```python
from build123d import *

# Parameters (mm, degrees)
F0_W          = 15.24
F0_H          = 15.24
F1_DEPTH      = 35.56
F2_R          = 3.175
F3_DEPTH      = 12.7
F3_DEPTH_BACK = 3.175
F4_R          = 3.175
F4_W          = 11.2
F4_H          = 5.9
F5_DEPTH      = 12.7
F6_T1_DEPTH   = 48.26
F7_R          = 3.302
F8_DEPTH      = 6.35


# Not quite as in the source:
# - a fillet or chamfer that OpenCascade refuses, or shapes differently, is made with other operations: its cross-section is extruded or revolved along the edge and cut away or added


with BuildPart() as f1:
    # F0 (on Top) → F1 (new body)
    with BuildSketch(Plane.XY):
        Rectangle(F0_W, F0_H)
    extrude(amount=F1_DEPTH)

    # F2 (on Front) → F3 (cut, two sides)
    with BuildSketch(Plane.XZ) as f3_sk:
        with Locations((0, 34.00425)):
            Circle(F2_R)
    extrude(amount=-F3_DEPTH, mode=Mode.SUBTRACT)
    extrude(f3_sk.sketch, amount=F3_DEPTH_BACK, mode=Mode.SUBTRACT)

    # F4 (on Right) → F5 (cut, symmetric)
    with BuildSketch(Plane.YZ):
        with Locations((0, 25.4)):
            Circle(F4_R)
        with Locations((0, 6.35)):
            Rectangle(F4_W, F4_H)
    extrude(amount=F5_DEPTH, both=True, mode=Mode.SUBTRACT)

    # F6: fillet of radius 2.54 on 4 edges, made by hand

    # F6_s2 → F6_t1 (cut)
    with BuildSketch(Plane.XY.offset(-6.35)):
        with BuildLine():
            ThreePointArc((7.62, 5.08), (6.8760512242, 6.8760512242), (5.08, 7.62))
            Line((5.08, 7.62), (7.62, 7.62))
            Line((7.62, 7.62), (7.62, 5.08))
        make_face()
        with BuildLine():
            ThreePointArc((5.08, -7.62), (6.8760512242, -6.8760512242), (7.62, -5.08))
            Line((7.62, -5.08), (7.62, -7.62))
            Line((7.62, -7.62), (5.08, -7.62))
        make_face()
        with BuildLine():
            ThreePointArc((-7.62, 5.08), (-6.8760512242, 6.8760512242), (-5.08, 7.62))
            Line((-5.08, 7.62), (-7.62, 7.62))
            Line((-7.62, 7.62), (-7.62, 5.08))
        make_face()
        with BuildLine():
            ThreePointArc((-5.08, -7.62), (-6.8760512242, -6.8760512242), (-7.62, -5.08))
            Line((-7.62, -5.08), (-7.62, -7.62))
            Line((-7.62, -7.62), (-5.08, -7.62))
        make_face()
    extrude(amount=F6_T1_DEPTH, mode=Mode.SUBTRACT)

    # F7 (on face) → F8 (cut)
    with BuildSketch(Plane(origin=(0, 0, 0), x_dir=(1, 0, 0), z_dir=(0, 0, -1))):
        Circle(F7_R)
    extrude(amount=-F8_DEPTH, mode=Mode.SUBTRACT)


solid = f1.part
```
Could you check a few things on this model? Use its own coordinates, in mm. A direction names the side the tool comes from. Round coordinates to 2 decimals unless told otherwise and drop trailing zeros. Loops run counter-clockwise (first coordinate to the right, second up) from the corner with the lowest first, then second, coordinate; pieces in that order, holes last. Notation, with made-up numbers: M -11,88.5 L 9,88.5 A7 cw 9,93.5 Z; hole C 37,-27.5 d7. An arc over 180 degrees is marked long. Put each result on its own line as item: value.
Q1. Imagine slicing it at C-C (x = -4.5). Write out the boundary of the cut face in (y, z) (3 decimals).
Check result:
outline: M -7.62,0 L 7.62,0 L 7.62,35.56 L -7.62,35.56 Z; hole M -5.6,3.4 L 5.6,3.4 L 5.6,9.3 L -5.6,9.3 Z; hole C 0,25.4 d6.35
Q2. Imagine slicing it at A-A (z = 25.4). Write out the boundary of the cut face in (x, y) (3 decimals), then the cut area to 3 significant figures.
Check result:
outline: M -7.62,-5.08 A2.54 ccw -5.08,-7.62 L 5.08,-7.62 A2.54 ccw 7.62,-5.08 L 7.62,-3.175 L -7.62,-3.175 Z; M -7.62,3.175 L 7.62,3.175 L 7.62,5.08 A2.54 ccw 5.08,7.62 L -5.08,7.62 A2.54 ccw -7.62,5.08 Z
area: 130 mm2
Q3. Thinking about a two-plate mould opening in Y: for faces 6 (the face through (-7.62, 1, 22)), 7 (the face through (-6.856, -6.896, 17.531)), 8 (the face through (0.11, -0.41, 28.55)), which applies, released by +Y, released by -Y, zero draft, split by the parting line, or undercut?
Check result:
face 6: zero draft
face 7: released by -Y
face 8: undercut
Q4. Imagine slicing it at B-B (x = 0). Write out the boundary of the cut face in (y, z) (3 decimals), then the cut area to 3 significant figures.
Check result:
outline: M -7.62,0 L -3.302,0 L -3.302,3.4 L -5.6,3.4 L -5.6,9.3 L 5.6,9.3 L 5.6,3.4 L 3.302,3.4 L 3.302,0 L 7.62,0 L 7.62,30.829 L -3.175,30.829 L -3.175,35.56 L -7.62,35.56 Z; hole C 0,25.4 d6.35
area: 371 mm2
Q5. On a 3-axis mill with a long thin cutter (end or side, diameter ignored), from which of +Z, -Z, +X, -X, +Y, -Y can I reach the whole of each face in a straight line? I mean faces 1 (the face through (3.5, -0.1, 3.4)), 2 (the face through (3.05, 1.26, 1.68)), 3 (the face through (-6.896, 6.856, 17.531)), 4 (the face through (6.856, -6.896, 17.531)), 5 (the face through (0, -3.175, 34)). Say none if no direction works.
Check result:
face 1: +X, -X
face 2: -Z
face 3: +Z, -Z, -X, +Y
face 4: +Z, -Z, +X, -Y
face 5: +Y
Q6. Imagine slicing it at D-D (z = 7). Write out the boundary of the cut face in (x, y).
Check result:
outline: M -7.57,-5.6 A2.54 ccw -5.08,-7.62 L 5.08,-7.62 A2.54 ccw 7.57,-5.6 Z; M -7.57,5.6 L 7.57,5.6 A2.54 ccw 5.08,7.62 L -5.08,7.62 A2.54 ccw Z
Q7. I need wall thicknesses on probe 1 along Y at (x, z) = (0, 1.75); probe 2 along Y at (x, z) = (-1.5, 25.4) (3 decimals); probe 3 along Z at (x, y) = (4.75, 4.75). Which ranges of each line are inside material? Lowest first, please.
Check result:
probe 1: -7.62 to -3.3, 3.3 to 7.62
probe 2: -7.62 to -3.175, 3.175 to 7.62
probe 3: 0 to 3.4, 9.3 to 35.56
Q8. For pin 1 (6 mm diameter, centred on x = -6, z = 29, fed in from +Y); pin 2 (1.4 mm diameter, centred on x = 1, z = 33.5, fed in from +Y) (3 decimals); pin 3 (5.5 mm diameter, centred on y = 0, z = 25.4, fed in from -X), each with a flat end and sliding along its axis, tell me the tip position at first contact or that it passes through.
Check result:
pin 1: y = 7.62
pin 2: y = -3.175
pin 3: through
